Check sheet for the drawn part. Datum: minimum x, y, z corner. Units: mm. A direction names the side the tool comes from. Give positions to 0.01 mm unless a question says otherwise; leave off trailing zeros. Loops run counter-clockwise (first coordinate to the right, second up) from the corner with the lowest first, then second, coordinate; pieces in that order, holes last. Notation, with made-up numbers: (55.25, -12) - (65.25, -12) arc R10 ccw to (65.25, -5) - close; hole circle Ø5 at (76, 8). An arc over 180 degrees is marked (long way). One line per item, written item: value. Start each with the question number.
1. Sectioned sample at C-C (x = 3). Record the cut outline in (y, z).
2. Sectioned sample at A-A (y = 2). Record the cut outline in (x, z) (1 decimal), plus the area to 3 significant figures.
3. Sectioned sample at D-D (y = 12.5). Record the cut outline in (x, z) (1 decimal), plus the area to 3 significant figures.
4. Scan lines: L1, parallel to Z at x = 17, y = 2.25; L2, parallel to Z at x = 29.5, y = 3 (1 decimal); L3, parallel to X at y = 3.25, z = 8.25. Record each from-to range of solid material in increasing order. Write a range as [from, to].
5. Access from +Z, -Z, +X, -X, +Y, -Y to the whole of each face (thin tool, end or side, straight path). Record for the marked faces 1, 2 and 3.
6. Sectioned sample at B-B (z = 15.5). Record the cut outline in (x, y) (1 decimal).
7. Gauge pin test, flat ends, axial feed: pin 1 (2.5 mm diameter, centred on y = 18.5, z = 4.5, fed in from +X); pin 2 (6 mm diameter, centred on x = 27, z = 9, fed in from -Y); pin 3 (9.5 mm diameter, centred on x = 25.5, z = 6.5, fed in from +Y). Record the tip position at first contact, or that the pin passes through.
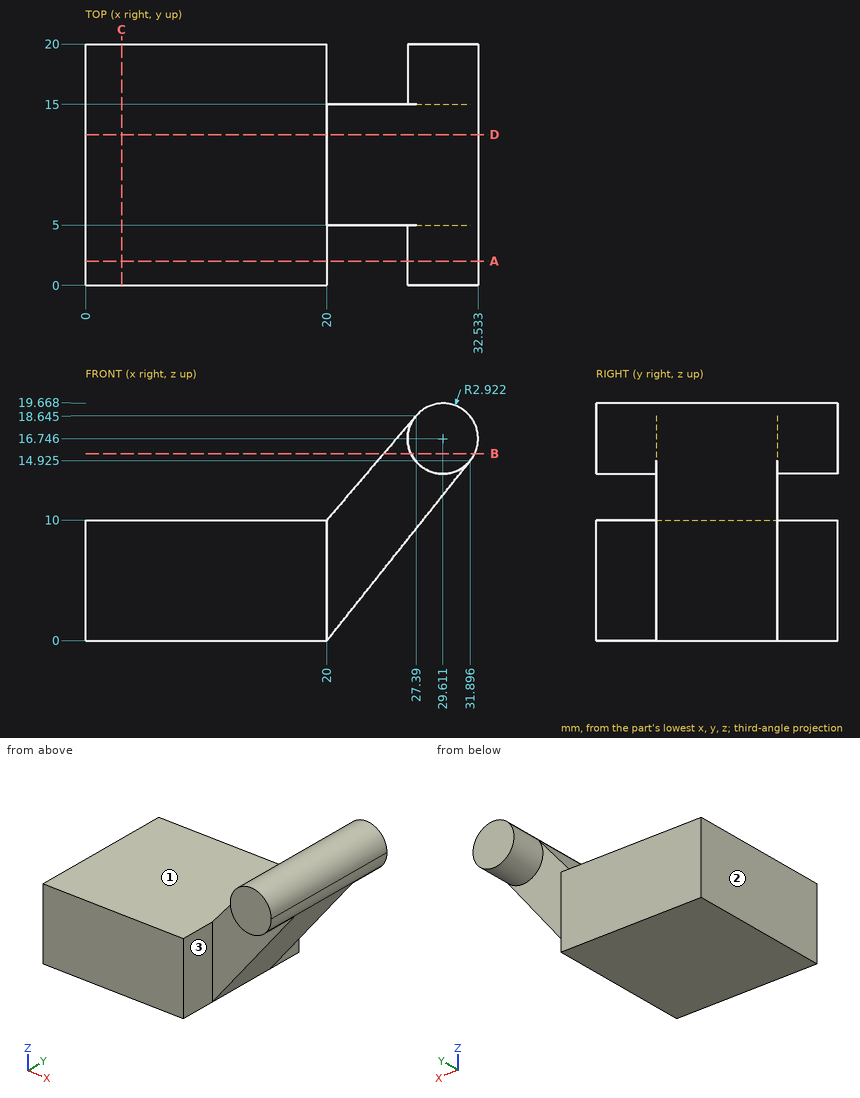
Results are:
1. outline: (0, 0) - (20, 0) - (20, 10) - (0, 10) - close
2. outline: (0, 0) - (20, 0) - (20, 10) - (0, 10) - close; (31.9, 14.9) arc R2.9 ccw to (32.5, 16.7) arc R2.9 ccw (long way) to start
2. area: 227 mm^2
3. outline: (0, 0) - (20, 0) - (31.9, 14.9) arc R2.9 ccw to (32.5, 16.7) arc R2.9 ccw to (27.4, 18.6) - (20, 10) - (0, 10) - close
3. area: 306 mm^2
4. L1: z = [0, 10]
4. L2: z = [13.8, 19.7]
4. L3: x = [0, 20]
5. face 1: +Z, -X, +Y, -Y
5. face 2: +Z, -Z, -X, +Y, -Y
5. face 3: +Z, -Z, +X, -Y
6. outline: (24.7, 5) - (27, 5) - (27, 0) - (32.3, 0) - (32.3, 20) - (27, 20) - (27, 15) - (24.7, 15) - close
7. pin 1: stops at x = 20
7. pin 2: stops at y = 5
7. pin 3: stops at y = 15
